Could you check a few things on this model? Use its own coordinates, in mm. A direction names the side the tool comes from. Coordinates: 2 decimals unless noted, no trailing zeros. Order: outer loops, then holes, each group sorted by start corner. A loop starts at its lowest first (then second) coordinate and runs counter-clockwise, first axis right, second up. Notation, with made-up numbers: M -5.5,-8.5 L 7.5,-8.5 A12 cw 7.5,-3.5 Z; hole C 25,51.5 d9. An arc over 180 degrees is marked long. One line per question, with ' | ' between items. Start each with the question number.
from build123d import *

# Parameters (mm, degrees)
SKETCH1_R           = 1.5
BOSS_EXTRUDE1_DEPTH = 10
FILLET1_R           = 1
FILLET2_R           = 1
FILLET3_R           = 1
FILLET4_R           = 1
FILLET5_R           = 1
FILLET6_R           = 1
FILLET7_R           = 1
FILLET8_R           = 1
SKETCH2_R           = 12.5
BOSS_EXTRUDE2_DEPTH = 2
SKETCH4_R           = 2.5
CUT_EXTRUDE1_DEPTH  = 10
SKETCH5_R           = 2.5
CUT_EXTRUDE2_DEPTH  = 50


with BuildPart() as part:
    # Sketch1 → Boss-Extrude1 (new body)
    with BuildSketch(Plane(origin=(0, 0, 0), x_dir=(1, 0, 0), z_dir=(0, 1, 0))):
        Polygon((37.3, 42.3), (5, 42.3), (0, 37.3), (0, 5), (5, 0), (37.3, 0), (42.3, 5), (42.3, 37.3), align=None)
        with Locations(Location((5, 5, 0), (0, 0, 270))):
            Circle(SKETCH1_R, mode=Mode.SUBTRACT)
        with Locations(Location((37.3, 5, 0), (0, 0, 270))):
            Circle(SKETCH1_R, mode=Mode.SUBTRACT)
        with Locations(Location((5, 37.3, 0), (0, 0, 270))):
            Circle(SKETCH1_R, mode=Mode.SUBTRACT)
        with Locations(Location((37.3, 37.3, 0), (0, 0, 270))):
            Circle(SKETCH1_R, mode=Mode.SUBTRACT)
    extrude(amount=BOSS_EXTRUDE1_DEPTH)

    # Fillet1
    fillet1_edges = [part.edges().sort_by_distance(p)[0] for p in [
        (0, 5, -5),
    ]]
    fillet(fillet1_edges, radius=FILLET1_R)

    # Fillet2
    fillet2_edges = [part.edges().sort_by_distance(p)[0] for p in [
        (5, 5, 0),
    ]]
    fillet(fillet2_edges, radius=FILLET2_R)

    # Fillet3
    fillet3_edges = [part.edges().sort_by_distance(p)[0] for p in [
        (37.3, 5, 0),
    ]]
    fillet(fillet3_edges, radius=FILLET3_R)

    # Fillet4
    fillet4_edges = [part.edges().sort_by_distance(p)[0] for p in [
        (42.3, 5, -5),
    ]]
    fillet(fillet4_edges, radius=FILLET4_R)

    # Fillet5
    fillet5_edges = [part.edges().sort_by_distance(p)[0] for p in [
        (42.3, 5, -37.3),
    ]]
    fillet(fillet5_edges, radius=FILLET5_R)

    # Fillet6
    fillet6_edges = [part.edges().sort_by_distance(p)[0] for p in [
        (37.3, 5, -42.3),
    ]]
    fillet(fillet6_edges, radius=FILLET6_R)

    # Fillet7
    fillet7_edges = [part.edges().sort_by_distance(p)[0] for p in [
        (5, 5, -42.3),
    ]]
    fillet(fillet7_edges, radius=FILLET7_R)

    # Fillet8
    fillet8_edges = [part.edges().sort_by_distance(p)[0] for p in [
        (0, 5, -37.3),
    ]]
    fillet(fillet8_edges, radius=FILLET8_R)

    # Sketch2 → Boss-Extrude2 (add)
    with BuildSketch(Plane.XZ):
        with Locations(Location((21.15, -21.15, 0), (0, 0, 90))):
            Circle(SKETCH2_R)
    extrude(amount=BOSS_EXTRUDE2_DEPTH)

    # Sketch4 → Cut-Extrude1 (cut)
    with BuildSketch(Plane.XZ.offset(2)):
        with Locations(Location((21.15, -21.15, 0), (0, 0, 270))):
            Circle(SKETCH4_R)
    extrude(amount=-CUT_EXTRUDE1_DEPTH, mode=Mode.SUBTRACT)

    # Sketch5 → Cut-Extrude2 (cut)
    with BuildSketch(Plane.XZ.offset(2)):
        with Locations(Location((21.15, -21.15, 0), (0, 0, 270))):
            Circle(SKETCH5_R)
    extrude(amount=-CUT_EXTRUDE2_DEPTH, mode=Mode.SUBTRACT)


solid = part.part
(1) If I drill on line 1 along X through (y, z) = (4.25, -21.15); line 2 along X through (y, z) = (3, -5); line 3 along Z through (x, y) = (38.5, 0.75), over which ranges is the centre line in solid material (lowest first)? Write a range as from..to.
(2) For P1, Ø1, axis at x = 10, z = -33.5, coming from the -Y side, with a flat end and sliding along its axis, tell me the tip position at first contact or that it passes through.
(3) Imagine slicing it at C-C, the plane x = 21.15. Write out the boundary of the cut face in (y, z).
(4) We'd pull the mould along X, two halves only. Please class faces 3 (the cylindrical face through (5.07, 4.93, -6.5)), 4 (the flat face through (39.8, 4.9, -2.5)), 5 (the flat face through (2.5, 4.9, -39.8)), 6 (the flat face through (26, 10, -21)): +X half, -X half, draft (parallel to the pull), parting line (faces both ways), or undercut.
(5) Imagine slicing it at A-A, the plane z = -21.15. Write out the boundary of the cut face in (x, y), plus the area to 3 significant figures.
(6) On a 3-axis mill with a long thin cutter (end or side, diameter ignored), from which of +Z, -Z, +X, -X, +Y, -Y can I reach the whole of each face in a straight line? I mean faces 1 (the cylindrical face through (17.395, -0.986, -9.227)), 2 (the cylindrical face through (5.07, 4.93, -38.8)). Say none if no direction works.
(7) Imagine slicing it at D-D, the plane z = -28. Write out the boundary of the cut face in (x, y), plus the area to 3 significant figures.
(8) Imagine slicing it at B-B, the plane y = 6.5. Write out the boundary of the cut face in (x, z).
Answers:
1) line 1: 0..18.65, 23.65..42.3 | line 2: 0.09..3.5, 6.5..35.8, 38.8..42.21 | line 3: -41.1..-38.2, -36.4..-5.9, -4.1..-1.2
2) P1: y = 0
3) outline: M -2,-33.65 L 0,-33.65 L 0,-42.3 L 10,-42.3 L 10,-23.65 L -2,-23.65 Z; M -2,-18.65 L 10,-18.65 L 10,0 L 0,0 L 0,-8.65 L -2,-8.65 Z
4) face 3: undercut | face 4: +X half | face 5: -X half | face 6: draft
5) outline: M 0,0 L 8.65,0 L 8.65,-2 L 18.65,-2 L 18.65,10 L 0,10 Z; M 23.65,-2 L 33.65,-2 L 33.65,0 L 42.3,0 L 42.3,10 L 23.65,10 Z | area: 413 mm²
6) face 1: -Y | face 2: +Y, -Y
7) outline: M 0,0 L 10.69,0 L 10.69,-2 L 31.61,-2 L 31.61,0 L 42.3,0 L 42.3,10 L 0,10 Z | area: 465 mm²
8) outline: M 0,-36.89 A1 ccw 0.29,-37.59 L 4.71,-42.01 A1 ccw 5.41,-42.3 L 36.89,-42.3 A1 ccw 37.59,-42.01 L 42.01,-37.59 A1 ccw 42.3,-36.89 L 42.3,-5.41 A1 ccw 42.01,-4.71 L 37.59,-0.29 A1 ccw 36.89,0 L 5.41,0 A1 ccw 4.71,-0.29 L 0.29,-4.71 A1 ccw 0,-5.41 Z; hole C 5,-37.3 d3; hole C 5,-5 d3; hole C 21.15,-21.15 d5; hole C 37.3,-37.3 d3; hole C 37.3,-5 d3
